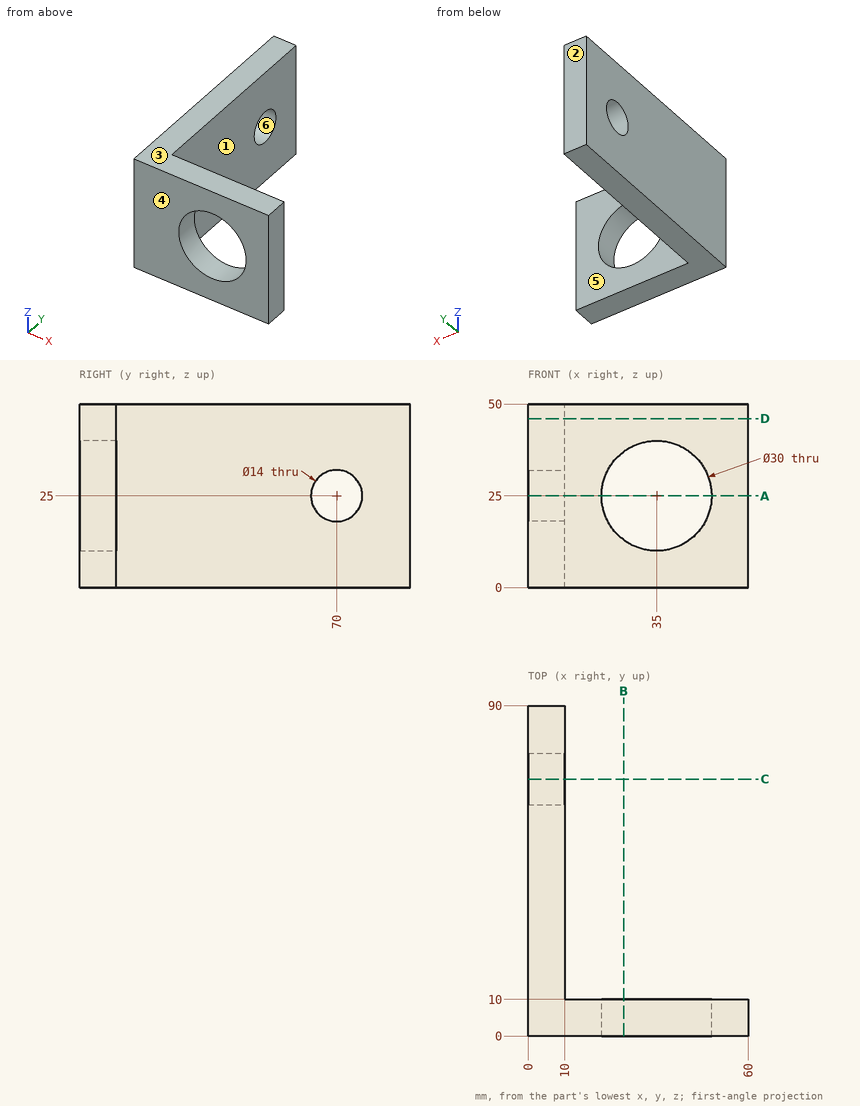
Geometry check sheet. Reference: drawing and pictorial views, mm from the part's lowest x, y, z. A direction names the side the tool comes from. Give positions to 0.01 mm unless a question says otherwise; leave off trailing zeros. Write each loop counter-clockwise with the first axis right and the second up, starting at its lowest first coordinate (ties: lowest second). Pieces come first, ordered by that corner, then holes. Notation, with made-up numbers: M -39.5,-18 L -7.5,-18 A12 ccw -7.5,-8 Z; hole C 76.5,43 d1. An arc over 180 degrees is marked long. Put each result on its own line as item: value. Start each with the question number.
1. Section check A-A (z = 25). Record the cut outline in (x, y), and give its area (3 significant figures).
2. Go/stop test with a flat-tipped pin: pin 1 Ø11 at (y, z) = (70, 25) entering from -X. Record where the tip stops, or that it passes through.
3. Draft check along Y on the marked faces 3, 4, 5 and 6. Enter one of: +Y half, -Y half, draft (parallel to the pull), parting line (faces both ways), or undercut.
4. Section check D-D (z = 46). Record the cut outline in (x, y).
5. Set-up check for the marked faces 1 and 2: record each of +Z, -Z, +X, -X, +Y, -Y from which the full face is reachable in a straight line by a thin tool's end or side.
6. Section check B-B (x = 26). Record the cut outline in (y, z).
7. Scan lines: line 1 along X through (y, z) = (5.5, 25); line 2 along Y through (x, z) = (6, 25); line 3 along Y through (x, z) = (39.5, 48.5). Record each from-to range of solid material in increasing order. Write a range as [from, to].
8. Section check C-C (y = 70). Record the cut outline in (x, z), and give its area (3 significant figures).
Answer list:
1. outline: M 0,0 L 20,0 L 20,10 L 10,10 L 10,63 L 0,63 Z; M 0,77 L 10,77 L 10,90 L 0,90 Z; M 50,0 L 60,0 L 60,10 L 50,10 Z
1. area: 960 mm2
2. pin 1: through
3. face 3: draft
3. face 4: -Y half
3. face 5: +Y half
3. face 6: undercut
4. outline: M 0,0 L 60,0 L 60,10 L 10,10 L 10,90 L 0,90 Z
5. face 1: +Z, -Z, +X, +Y
5. face 2: +Z, -Z, +X, -X, +Y
6. outline: M 0,0 L 10,0 L 10,13 L 0,13 Z; M 0,37 L 10,37 L 10,50 L 0,50 Z
7. line 1: [0, 20], [50, 60]
7. line 2: [0, 63], [77, 90]
7. line 3: [0, 10]
8. outline: M 0,0 L 10,0 L 10,18 L 0,18 Z; M 0,32 L 10,32 L 10,50 L 0,50 Z
8. area: 360 mm2
